Source: CAD feature listing. Evaluate the final solid. Frame: model axes, mm. Give positions to 0.01 mm unless a question says otherwise; leave off trailing zeros. Loops run counter-clockwise (first coordinate to the right, second up) from the corner with the lowest first, then second, coordinate; pieces in that order, holes last. Notation, with made-up numbers: (57, 2) -> (99, 2) arc R18 cw to (99, 6) -> close; hole circle Ø1 at (46.25, 64). An arc over 180 degrees is marked (long way). Put each result on its own line as item: value.
```python
from build123d import *

# Parameters (mm, degrees)
F0_W     = 56.4
F0_H     = 40
F0_R     = 2.25
F0_R_2   = 2.55
F1_DEPTH = 5


with BuildPart() as f1:
    # F0 (on Top) → F1 (new body)
    with BuildSketch(Plane.XY):
        with Locations((0, 48.2)):
            Rectangle(F0_W, F0_H)
        with Locations((-18.2, 38.2)):
            Circle(F0_R, mode=Mode.SUBTRACT)
        with Locations((18.2, 38.2)):
            Circle(F0_R, mode=Mode.SUBTRACT)
        with Locations((-18.2, 58.2)):
            Circle(F0_R, mode=Mode.SUBTRACT)
        with BuildLine():
            Line((28.2, 28.2), (-28.2, 28.2))
            Line((-28.2, 28.2), (-28.2, 13.2))
            Line((-28.2, 13.2), (-14.353048, 13.2))
            ThreePointArc((-14.353048, 13.2), (0, 19.5), (14.353048, 13.2))
            Line((14.353048, 13.2), (28.2, 13.2))
            Line((28.2, 13.2), (28.2, 28.2))
        make_face()
        with Locations((-23.57, 23.57)):
            Circle(F0_R_2, mode=Mode.SUBTRACT)
        with Locations((23.57, 23.57)):
            Circle(F0_R_2, mode=Mode.SUBTRACT)
    extrude(amount=F1_DEPTH)


solid = f1.part
```
(1) Draft query along Y for faces 1 (the flat face through (0, 41, 0)), 2 (the cylindrical face through (23.02, 21.08, 2.46)), 3 (the flat face through (0, 68.2, 2)). Return one class per face: released by +Y, released by -Y, zero draft, split by the parting line, or undercut.
Calculated:
face 1: zero draft
face 2: undercut
face 3: released by +Y
(2) Section C-C on x = 23.57. Return loops of the section in (y, z).
Calculated:
outline: (13.2, 0) -> (21.02, 0) -> (21.02, 5) -> (13.2, 5) -> close; (26.12, 0) -> (68.2, 0) -> (68.2, 5) -> (26.12, 5) -> close
(3) Section B-B on x = -18.2. Return loops of the section in (y, z), then the cut area to 3 significant figures.
Calculated:
outline: (13.2, 0) -> (35.95, 0) -> (35.95, 5) -> (13.2, 5) -> close; (40.45, 0) -> (55.95, 0) -> (55.95, 5) -> (40.45, 5) -> close; (60.45, 0) -> (68.2, 0) -> (68.2, 5) -> (60.45, 5) -> close
area: 230 mm²
(4) Section D-D on y = 38.2. Return loops of the section in (x, z), then the cut area to 3 significant figures.
Calculated:
outline: (-28.2, 0) -> (-20.45, 0) -> (-20.45, 5) -> (-28.2, 5) -> close; (-15.95, 0) -> (15.95, 0) -> (15.95, 5) -> (-15.95, 5) -> close; (20.45, 0) -> (28.2, 0) -> (28.2, 5) -> (20.45, 5) -> close
area: 237 mm²
(5) Section A-A on z = 1.45. Return loops of the section in (x, y), then the cut area to 3 significant figures.
Calculated:
outline: (-28.2, 13.2) -> (-14.35, 13.2) arc R19.5 cw to (14.35, 13.2) -> (28.2, 13.2) -> (28.2, 68.2) -> (-28.2, 68.2) -> close; hole circle Ø5.1 at (-23.57, 23.57); hole circle Ø4.5 at (-18.2, 38.2); hole circle Ø4.5 at (-18.2, 58.2); hole circle Ø4.5 at (18.2, 38.2); hole circle Ø5.1 at (23.57, 23.57)
area: 2,890 mm²
(6) Line query: probe 1 along Y at (x, z) = (23.57, 1.15); probe 2 along X at (y, z) = (39, 3.8); probe 3 along X at (y, z) = (25, 1.45). Output: solid intervals per line, ascending. Write a range as from..to.
Calculated:
probe 1: y = 13.2..21.02, 26.12..68.2
probe 2: x = -28.2..-20.3, -16.1..16.1, 20.3..28.2
probe 3: x = -28.2..-25.68, -21.46..21.46, 25.68..28.2
(7) First-contact query: P1, Ø5, axis at x = -18.2, y = 58.2, coming from the -Z side; P2, Ø1, axis at x = -6, z = 4, coming from the -Y side. Flat tips, straight axial feed; report the tip coordinate or a pass-through.
Calculated:
P1: stops at z = 0
P2: stops at y = 18.38
